Can you work these out from the drawing? Everything is in mm from the part's minimum corner. A direction names the side the tool comes from. Round coordinates to 2 decimals unless told otherwise and drop trailing zeros. Loops run counter-clockwise (first coordinate to the right, second up) from the corner with the lowest first, then second, coordinate; pieces in that order, holes last. Notation, with made-up numbers: M -9.75,49.25 L 24.25,49.25 A20 cw 24.25,66.25 Z; hole C 81,83 d8. An arc over 180 degrees is marked long. Use a Markdown table: item, result.
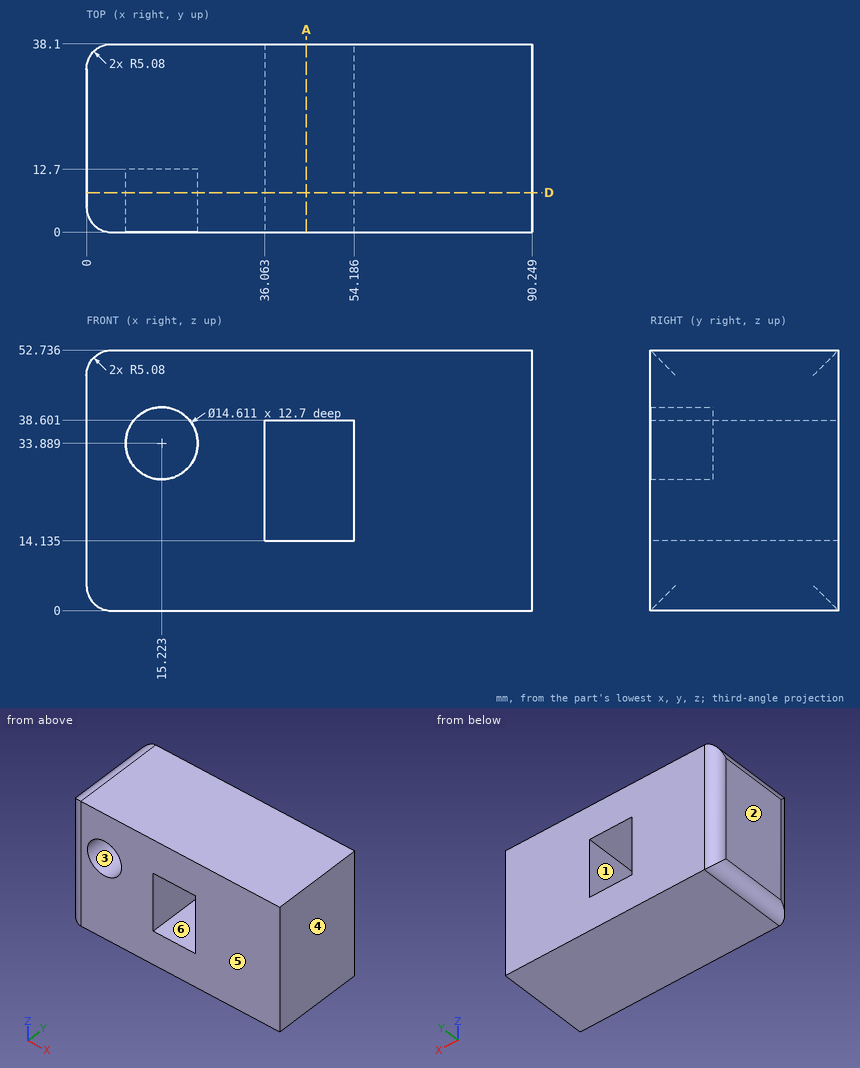
1. Imagine slicing it at D-D, the plane y = 8. State how many separate pieces and enclosed holes the cut face has, then the cut area to 3 significant figures.
Answer sheet:
| item | result |
|---|---|
| separate pieces | 1 |
| enclosed holes | 2 |
| area | 4,140 mm2 |
2. Imagine slicing it at A-A, the plane x = 44.5. Write out the boundary of the cut face in (y, z) (1 decimal).
Answer sheet:
| item | result |
|---|---|
| outline | M 0,0 L 38.1,0 L 38.1,14.1 L 0,14.1 Z; M 0,38.6 L 38.1,38.6 L 38.1,52.7 L 0,52.7 Z |
3. We'd pull the mould along X, two halves only. Please class the marked faces 4, 5 and 6: +X half, -X half, draft (parallel to the pull), parting line (faces both ways), or undercut.
Answer sheet:
| item | result |
|---|---|
| face 4 | +X half |
| face 5 | draft |
| face 6 | undercut |
4. Which directions (+Z, -Z, +X, -X, +Y, -Y) give clear straight access to the entire face, cutting with the end or side of a thin tool? Please do the marked faces 1, 2 and 3.
Answer sheet:
| item | result |
|---|---|
| face 1 | +Y, -Y |
| face 2 | +Z, -Z, -X, +Y, -Y |
| face 3 | -Y |
5. I need wall thicknesses on probe 1 along Z at (x, y) = (47.5, 4) (1 decimal); probe 2 along X at (y, z) = (5, 45). Which ranges of each line are inside material? Lowest first, please. Write a range as from..to.
Answer sheet:
| item | result |
|---|---|
| probe 1 | 0..14.1, 38.6..52.7 |
| probe 2 | 0..90.25 |
